from build123d import *

# Parameters (mm, degrees)
ESQUISSE1_W                           = 26.253582595
ESQUISSE1_H                           = 55
BOSS_EXTRU_1_DEPTH                    = 5
BOSS_EXTRU_2_DEPTH                    = 5
BOSS_EXTRU_3_DEPTH                    = 5
ENL_V_MAT_EXTRU_1_DEPTH               = 5
ESQUISSE5_W                           = 5
ESQUISSE5_H                           = 50
BOSS_EXTRU_4_DEPTH                    = 36.246417405
BOSS_EXTRU_5_DEPTH                    = 5
BOSS_EXTRU_6_DEPTH                    = 5
BOSS_EXTRU_7_DEPTH                    = 5
DIAM_TRE_DU_PER_AGE_12_2_12_2_1_D     = 12.2
DIAM_TRE_DU_PER_AGE_12_2_12_2_1_DEPTH = 5
DIAM_TRE_DU_PER_AGE_3_2_3_2_1_D       = 3.2
CONG_1_R                              = 1.6
ESQUISSE13_W                          = 9.997056275
ESQUISSE13_H                          = 5
ESQUISSE13_W_2                        = 2.945778535
ESQUISSE13_W_3                        = 2.95
ESQUISSE13_W_4                        = 5
ESQUISSE13_H_2                        = 2.95
BOSS_EXTRU_8_DEPTH                    = 5
ENL_V_MAT_EXTRU_2_DEPTH               = 5
CHANFREIN1_SIZE                       = 2


with BuildPart() as part:
    # Esquisse1 → Boss.-Extru.1 (new body)
    with BuildSketch(Plane(origin=(0, 0, 0), x_dir=(-1, 0, 0), z_dir=(0, 0, -1))):
        with Locations((-18.123208703, 2.5)):
            Rectangle(ESQUISSE1_W, ESQUISSE1_H)
    extrude(amount=-BOSS_EXTRU_1_DEPTH)

    # Esquisse2 → Boss.-Extru.2 (add)
    with BuildSketch(Plane(origin=(31.25, 0, 0), x_dir=(0, 0, -1), z_dir=(1, 0, 0))):
        Polygon((0, 15), (-2.05, 15), (-5, 17.95), (-5, 30), (0, 30), align=None)
    extrude(amount=BOSS_EXTRU_2_DEPTH)

    # Esquisse3 → Boss.-Extru.3 (add)
    with BuildSketch(Plane(origin=(31.25, 0, 0), x_dir=(0, 0, -1), z_dir=(1, 0, 0))):
        Polygon((-5, -12.95), (-2.05, -10), (0, -10), (0, -25), (-5, -25), align=None)
    extrude(amount=BOSS_EXTRU_3_DEPTH)

    # Esquisse4 → Enlèv. mat.-Extru.1 (cut)
    with BuildSketch(Plane(origin=(0, 30, 0), x_dir=(-1, 0, 0), z_dir=(0, 1, 0))):
        Polygon((-4.996417405, 5), (-7.946417405, 5), (-4.996417405, 2.05), align=None)
    extrude(amount=-ENL_V_MAT_EXTRU_1_DEPTH, mode=Mode.SUBTRACT)

    # Esquisse5 → Boss.-Extru.4 (add)
    with BuildSketch(Plane.ZY.offset(-4.996417405)):
        with Locations((2.5, 0)):
            Rectangle(ESQUISSE5_W, ESQUISSE5_H)
    extrude(amount=BOSS_EXTRU_4_DEPTH)

    # Esquisse6 → Boss.-Extru.5 (add)
    with BuildSketch(Plane.ZY.offset(31.25)):
        Polygon((0, -25), (0, -10), (2.05, -10), (5, -12.95), (5, -25), align=None)
    extrude(amount=BOSS_EXTRU_5_DEPTH)

    # Esquisse7 → Boss.-Extru.6 (add)
    with BuildSketch(Plane.ZY.offset(31.25)):
        Polygon((0, 25), (5, 25), (5, 17.95), (2.05, 15), (0, 15), align=None)
    extrude(amount=BOSS_EXTRU_6_DEPTH)

    # Esquisse8 → Boss.-Extru.7 (add)
    with BuildSketch(Plane(origin=(0, 25, 0), x_dir=(-1, 0, 0), z_dir=(0, 1, 0))):
        Polygon((5.00063887, 2.054221466), (7.946417405, 5), (36.25, 5), (36.25, 0), (5.00063887, 0), align=None)
    extrude(amount=BOSS_EXTRU_7_DEPTH)

    # Diamètre du perçage Ø12.2 (12.2)1
    with Locations(Plane.XY.offset(5)):
        with Locations((0, -7)):
            Hole(DIAM_TRE_DU_PER_AGE_12_2_12_2_1_D / 2, depth=DIAM_TRE_DU_PER_AGE_12_2_12_2_1_DEPTH)

    # Diamètre du perçage Ø3.2 (3.2)1 (through all)
    with Locations(Plane.XY.offset(5)):
        with Locations((-7.75, -13.423393759), (15.5, 0), (-7.75, 13.423393759), (7.75, 13.423393759), (7.75, -13.423393759), (-15.5, 0)):
            Hole(DIAM_TRE_DU_PER_AGE_3_2_3_2_1_D / 2)

    # Congé1
    cong_1_edges = [part.edges().sort_by_distance(p)[0] for p in [
        (-5.00063887, 27.5, 2.054221466),
        (33.75, 15, 2.05),
        (33.75, -10, 2.05),
        (4.996417405, 27.5, 2.05),
        (-33.75, -10, 2.05),
        (-33.75, 15, 2.05),
    ]]
    fillet(cong_1_edges, radius=CONG_1_R)

    # Esquisse13 → Boss.-Extru.8 (add)
    with BuildSketch(Plane.XY.offset(5)):
        with Locations((-0.002110733, 27.5)):
            Rectangle(ESQUISSE13_W, ESQUISSE13_H)
        with Locations((-6.473528138, 27.5)):
            Rectangle(ESQUISSE13_W_2, ESQUISSE13_H)
        with Locations((6.471417405, 27.5)):
            Rectangle(ESQUISSE13_W_3, ESQUISSE13_H)
        with Locations((33.75, 16.475)):
            Rectangle(ESQUISSE13_W_4, ESQUISSE13_H_2)
        with Locations((33.75, -11.475)):
            Rectangle(ESQUISSE13_W_4, ESQUISSE13_H_2)
        with Locations((-33.75, -11.475)):
            Rectangle(ESQUISSE13_W_4, ESQUISSE13_H_2)
        with Locations((-33.75, 16.475)):
            Rectangle(ESQUISSE13_W_4, ESQUISSE13_H_2)
    extrude(amount=-BOSS_EXTRU_8_DEPTH)

    # Esquisse14 → Enlèv. mat.-Extru.2 (cut)
    with BuildSketch(Plane.XY.offset(5)):
        Polygon((-1.55, 19), (1.55, 19), (1.55, 22), (2.78, 22), (2.78, 25), (1.55, 25), (1.55, 30), (-1.55, 30), (-1.55, 25), (-2.77, 25), (-2.77, 22), (-1.55, 22), align=None)
        Polygon((-23.25, 0.95), (-20.25, 0.95), (-20.25, 4.05), (-23.25, 4.05), (-23.25, 5.27), (-26.25, 5.27), (-26.25, 4.05), (-31.25, 4.05), (-31.25, 0.95), (-26.25, 0.95), (-26.25, -0.28), (-23.25, -0.28), align=None)
        Polygon((23.25, -0.28), (26.25, -0.28), (26.25, 0.95), (31.25, 0.95), (31.25, 4.05), (26.25, 4.05), (26.25, 5.27), (23.25, 5.27), (23.25, 4.05), (20.25, 4.05), (20.25, 0.95), (23.25, 0.95), align=None)
        Polygon((-1.55, -17), (-2.77, -17), (-2.77, -20), (-1.55, -20), (-1.55, -25), (1.55, -25), (1.55, -20), (2.78, -20), (2.78, -17), (1.55, -17), (1.55, -14), (-1.55, -14), align=None)
    extrude(amount=-ENL_V_MAT_EXTRU_2_DEPTH, mode=Mode.SUBTRACT)

    # Chanfrein1
    chanfrein1_edges = [part.edges().sort_by_distance(p)[0] for p in [
        (-13.9, 0, 5),
        (9.35, -13.423393759, 5),
        (9.35, 13.423393759, 5),
        (-6.15, 13.423393759, 5),
        (17.1, 0, 5),
        (-6.15, -13.423393759, 5),
    ]]
    chamfer(chanfrein1_edges, length=CHANFREIN1_SIZE)


solid = part.part
Input: part model. Units: mm. Frame: model coordinates. A direction names the side the tool comes from. Coordinates: 2 decimals unless noted, no trailing zeros. Order: outer loops, then holes, each group sorted by start corner. A loop starts at its lowest first (then second) coordinate and runs counter-clockwise, first axis right, second up. Notation, with made-up numbers: M -32.5,31 L -3.5,31 A22 ccw -3.5,63 Z; hole C 84,86 d11. An arc over 180 degrees is marked long. Answer as CSV lines item,"result".
1. Section B-B (y = 24). Return the cut outline in (x, z).
Reported:
outline,"M -36.25,0 L -2.77,0 L -2.77,5 L -36.25,5 Z; M 2.78,0 L 36.25,0 L 36.25,5 L 2.78,5 Z"
2. Section C-C (x = -7.75). Return the cut outline in (y, z).
Reported:
outline,"M -25,0 L -15.02,0 L -15.02,3 L -17.02,5 L -25,5 Z; M -11.82,0 L 11.82,0 L 11.82,3 L 9.82,5 L -9.82,5 L -11.82,3 Z; M 15.02,0 L 30,0 L 30,5 L 17.02,5 L 15.02,3 Z"
3. First-contact query: P1, Ø2, axis at y = -6.5, z = 1.5, coming from the -X side; P2, Ø4, axis at x = -7.75, y = 13.42, coming from the +Z side; P3, Ø1.5, axis at y = -6, z = 3, coming from the +X side; P4, Ø3, axis at x = -7.75, y = -13.42, coming from the -Z side. Flat tips, straight axial feed; report the tip coordinate or a pass-through.
Reported:
P1,"x = -31.25"
P2,"z = 3.4"
P3,"x = 31.25"
P4,"through"
4. Access query for faces 1 (the flat face through (1.55, -16, 3)), 2 (the flat face through (22, 4.05, 3)), 3 (the flat face through (-20.25, 2, 3)), 4 (the flat face through (-2.77, -18, 3)), 5 (the flat face through (0, 19, 3)). Directions: +Z, -Z, +X, -X, +Y, -Y. A direction counts if a zero-diameter tool reaches every point of the face in a straight line with its end or side. Return the directions, or none.
Reported:
face 1,"+Z, -Z, -Y"
face 2,"+Z, -Z, +X"
face 3,"+Z, -Z, -X"
face 4,"+Z, -Z"
face 5,"+Z, -Z, +Y"
5. Material intervals for line 1 (X direction, y = 5, z = 2.15); line 2 (X direction, y = -16, z = 0.75); line 3 (Y direction, x = 7.75, z = 1.2), sorted ascending. Write a range as from..to.
Reported:
line 1,"-31.25..-26.25, -23.25..23.25, 26.25..31.25"
line 2,"-36.25..-1.55, 1.55..36.25"
line 3,"-25..-15.02, -11.82..11.82, 15.02..30"
6. Section A-A (x = 0). Return the cut outline in (y, z), then the cut area to 3 significant figures.
Reported:
outline,"M -14,0 L -13.1,0 L -13.1,5 L -14,5 Z; M -0.9,0 L 19,0 L 19,5 L -0.9,5 Z"
area,"104 mm2"
7. Pull-direction query (X, two-part tool) for faces 6 (the cylindrical face through (-6.571, 14.505, 1.479)), 7 (the flat face through (-36.25, -17, 3)), 8 (the flat face through (1.55, 20, 3)), 9 (the flat face through (29, 4.05, 3)); classes: released by +X, released by -X, zero draft, split by the parting line, or undercut.
Reported:
face 6,"undercut"
face 7,"released by -X"
face 8,"undercut"
face 9,"zero draft"
8. Section D-D (x = 15.5). Return the cut outline in (y, z).
Reported:
outline,"M -25,0 L -1.6,0 L -1.6,3 L -3.6,5 L -25,5 Z; M 1.6,0 L 30,0 L 30,5 L 3.6,5 L 1.6,3 Z"
